Model file for the job. Use its own axes, mm. A direction names the side the tool comes from. Coordinates: 2 decimals unless noted, no trailing zeros. Loops run counter-clockwise (first coordinate to the right, second up) from the corner with the lowest first, then second, coordinate; pieces in that order, holes last. Notation, with made-up numbers: (-11.5, 8) -> (26.5, 8) arc R16 cw to (26.5, 32) -> close; hole circle Ø1 at (78, -31). An arc over 180 degrees is marked (long way). Use one line per item in the form item = value.
```python
from build123d import *

# Parameters (mm, degrees)
BOSS_EXTRUDE1_DEPTH           = 2.5
SKETCH2_W                     = 7
SKETCH2_H                     = 2.5
BOSS_EXTRUDE2_DEPTH           = 9.5
CUT_EXTRUDE1_DEPTH            = 9.5
SKETCH4_R                     = 1.25
CUT_EXTRUDE2_DEPTH            = 9.5
CBORE_FOR_M2_SHCS1_AT_2_COUNT = 2
CBORE_FOR_M2_SHCS1_AT_2_PITCH = 10
SKETCH8_R                     = 2.2
CUT_EXTRUDE3_DEPTH            = 9.5
SKETCH11_W                    = 19.05
SKETCH11_H                    = 19.05
BOSS_EXTRUDE3_DEPTH           = 5
FILLET1_R                     = 0.07


with BuildPart() as part:
    # Sketch1 → Boss-Extrude1 (new body, symmetric)
    with BuildSketch(Plane(origin=(0, 0, 0), x_dir=(1, 0, 0), z_dir=(0, 1, 0))):
        with BuildLine():
            Line((1.95, 0), (7.9492, 0))
            ThreePointArc((7.9492, 0), (0, -7.9492), (-7.9492, 0))
            Line((-7.9492, 0), (-1.95, 0))
            ThreePointArc((-1.95, 0), (0, -1.95), (1.95, 0))
        make_face()
    extrude(amount=BOSS_EXTRUDE1_DEPTH, both=True)

    # Sketch2 → Boss-Extrude2 (add)
    with BuildSketch(Plane(origin=(0, 2.5, 0), x_dir=(1, 0, 0), z_dir=(0, 1, 0))):
        with Locations((0, -5)):
            Rectangle(SKETCH2_W, SKETCH2_H)
    extrude(amount=BOSS_EXTRUDE2_DEPTH)

    # Sketch3 → Cut-Extrude1 (cut)
    with BuildSketch(Plane(origin=(0, 0, 3.75), x_dir=(-1, 0, 0), z_dir=(0, 0, -1))):
        with BuildLine():
            Line((-3.5, 8.5), (-3.5, 14.886359519))
            Line((-3.5, 14.886359519), (0, 16.809201746))
            Line((0, 16.809201746), (3.5, 14.5))
            Line((3.5, 14.5), (3.5, 8.5))
            ThreePointArc((3.5, 8.5), (0, 12), (-3.5, 8.5))
        make_face()
    extrude(amount=-CUT_EXTRUDE1_DEPTH, mode=Mode.SUBTRACT)

    # Sketch4 → Cut-Extrude2 (cut)
    with BuildSketch(Plane(origin=(0, 0, 3.75), x_dir=(-1, 0, 0), z_dir=(0, 0, -1))):
        with Locations((0, 8.5)):
            Circle(SKETCH4_R)
    extrude(amount=-CUT_EXTRUDE2_DEPTH, mode=Mode.SUBTRACT)

    # Sketch7 → CBORE for M2 SHCS1 (revolve, cut)
    with BuildSketch(Plane(origin=(5, 0, 7), x_dir=(0, -1, 0), z_dir=(1, 0, 0))):
        Polygon((0, 0), (0, 7), (1.2, 7), (1.2, 2), (2.2, 2), (2.2, 0), align=None)
    cbore_for_m2_shcs1 = revolve(axis=Axis((5, 0, 13.35), (0, 0, -1)), mode=Mode.SUBTRACT)

    # CBORE for M2 SHCS1 at 2: CBORE for M2 SHCS1 ×2
    with Locations(*[(-i * CBORE_FOR_M2_SHCS1_AT_2_PITCH, 0, 0) for i in range(1, CBORE_FOR_M2_SHCS1_AT_2_COUNT)]):
        add(cbore_for_m2_shcs1, mode=Mode.SUBTRACT)

    # Sketch8 → Cut-Extrude3 (cut)
    with BuildSketch(Plane(origin=(0, 0, 7), x_dir=(-1, 0, 0), z_dir=(0, 0, -1))):
        with Locations((-5, 0)):
            Circle(SKETCH8_R)
        with Locations((5, 0)):
            Circle(SKETCH8_R)
    extrude(amount=-CUT_EXTRUDE3_DEPTH, mode=Mode.SUBTRACT)

    # Sketch11 → Boss-Extrude3 (add)
    with BuildSketch(Plane.XZ.offset(2.5)):
        with Locations((0, 4)):
            Rectangle(SKETCH11_W, SKETCH11_H)
    extrude(amount=BOSS_EXTRUDE3_DEPTH)

    # Fillet1
    fillet1_edges = [part.edges().sort_by_distance(p)[0] for p in [
        (1.95, 0, 0),
        (-1.95, 0, 0),
    ]]
    fillet(fillet1_edges, radius=FILLET1_R)


solid = part.part
```
Q1. Band-saw the part on C-C, the plane y = 4.75. Write the cut outline in (x, z), and give its area (3 significant figures).
Result:
outline = (-3.5, 3.75) -> (3.5, 3.75) -> (3.5, 6.25) -> (-3.5, 6.25) -> close
area = 17.5 mm2
Q2. Which spindle directions (+Z, -Z, +X, -X, +Y, -Y) get a long thin tool onto all of the face, cutting with end or side? Do faces 5 (the face through (-3.5, 5, 5)), 6 (the face through (3.5, 5, 5)), 7 (the face through (0, 7, 3.75)), 8 (the face through (-0.04, 0.04, 1.95)). Say none if no direction does.
Result:
face_5 = +Z, -Z, -X, +Y
face_6 = +Z, -Z, +X, +Y
face_7 = -Z, +X, -X, +Y
face_8 = -Z, +Y
Q3. Band-saw the part on D-D, the plane x = 7. Write the cut outline in (y, z) (3 decimals), and give its area (3 significant figures).
Result:
outline = (-7.5, -5.525) -> (-2.5, -5.525) -> (-2.5, 0) -> (2.5, 0) -> (2.5, 3.767) -> (-2.5, 3.767) -> (-2.5, 13.525) -> (-7.5, 13.525) -> close
area = 114 mm2
Q4. Band-saw the part on A-A, the plane x = 5. Write the cut outline in (y, z) (3 decimals), and give its area (3 significant figures).
Result:
outline = (-7.5, -5.525) -> (-2.5, -5.525) -> (-2.5, 0) -> (-1.2, 0) -> (-1.2, 5) -> (-2.2, 5) -> (-2.2, 6.18) -> (-2.5, 6.18) -> (-2.5, 13.525) -> (-7.5, 13.525) -> close; (1.2, 0) -> (2.5, 0) -> (2.5, 6.18) -> (2.2, 6.18) -> (2.2, 5) -> (1.2, 5) -> close
area = 109 mm2
Q5. Pin check, flat tips, straight feed: pin 1 Ø4 at (x, y) = (-2.5, 3.5) entering from +Z; pin 2 Ø2 at (y, z) = (6.5, 4.5) entering from -X; pin 3 Ø3 at (y, z) = (3, -2.5) entering from -X; pin 4 Ø2 at (x, y) = (0.5, 8.5) entering from -Z. Stop position of each tip, or through.
Result:
pin_1 = 7.91
pin_2 = -3.5
pin_3 = through
pin_4 = 3.75
Q6. Band-saw the part on B-B, the plane x = 0. Write the cut outline in (y, z) (3 decimals).
Result:
outline = (-7.5, -5.525) -> (-2.5, -5.525) -> (-2.5, 1.95) -> (2.5, 1.95) -> (2.5, 3.75) -> (7.25, 3.75) -> (7.25, 6.25) -> (2.5, 6.25) -> (2.5, 7.949) -> (-2.5, 7.949) -> (-2.5, 13.525) -> (-7.5, 13.525) -> close; (9.75, 3.75) -> (12, 3.75) -> (12, 6.25) -> (9.75, 6.25) -> close
Q7. Mould opens along Y. For faces 1 (the face through (0, 12, 5)), 2 (the face through (0, -7.5, 4)), 3 (the face through (-4, 1, 0)), 4 (the face through (-4, -1, 5)) say: released by +Y, released by -Y, zero draft, split by the parting line, or undercut.
Result:
face_1 = released by +Y
face_2 = released by -Y
face_3 = zero draft
face_4 = undercut
Q8. Wall check: line 1 along Y through (x, z) = (0, 4.75); line 2 along Y through (x, z) = (-5, 3.15); line 3 along Y through (x, z) = (-2.75, -2). Give the ranges that are in metal, low to high.
Result:
line_1 = -7.5 to 7.25, 9.75 to 12
line_2 = -7.5 to -1.2, 1.2 to 2.5
line_3 = -7.5 to -2.5
